Part model, mm, in its own coordinate system. Face numbers are marked on the shaded views. A direction names the side the tool comes from. Give positions to 0.01 mm unless a question says otherwise; leave off trailing zeros. Loops run counter-clockwise (first coordinate to the right, second up) from the corner with the lowest first, then second, coordinate; pieces in that order, holes last. Notation, with made-up numbers: (-22, -17.5) -> (-12, -17.5) arc R19 cw to (-12, 10.5) -> close; hole circle Ø1 at (-21, 45.5). An arc over 180 degrees is marked (long way). One line per question, with ' | ' between items.
```python
from build123d import *

# Parameters (mm, degrees)
F1_DEPTH = 19.05
F2_W     = 44.45
F2_H     = 63.5
F3_DEPTH = 19.05
F4_W     = 44.45
F4_H     = 19.05
F5_DEPTH = 12.7


with BuildPart() as f1:
    # F0 (on Top) → F1 (new body)
    with BuildSketch(Plane.XY):
        Polygon((0, 12.7), (0, 0), (63.5, 0), (63.5, 44.45), (44.45, 44.45), align=None)
    extrude(amount=F1_DEPTH)

    # F2 (on Front) → F3 (join)
    with BuildSketch(Plane.XZ):
        with Locations((41.275, -31.75)):
            Rectangle(F2_W, F2_H)
    extrude(amount=-F3_DEPTH)

    # F4 (on face) → F5 (join)
    with BuildSketch(Plane(origin=(0, 0, -63.5), x_dir=(1, 0, 0), z_dir=(0, 0, -1))):
        Polygon((19.05, 0), (0, 0), (0, -12.8343682736), (44.5106774569, -44.7837524116), (63.5, -44.7837524116), (63.5, -19.05), (19.05, -19.05), align=None)
        with Locations((41.275, -9.525)):
            Rectangle(F4_W, F4_H)
    extrude(amount=F5_DEPTH)


solid = f1.part
```
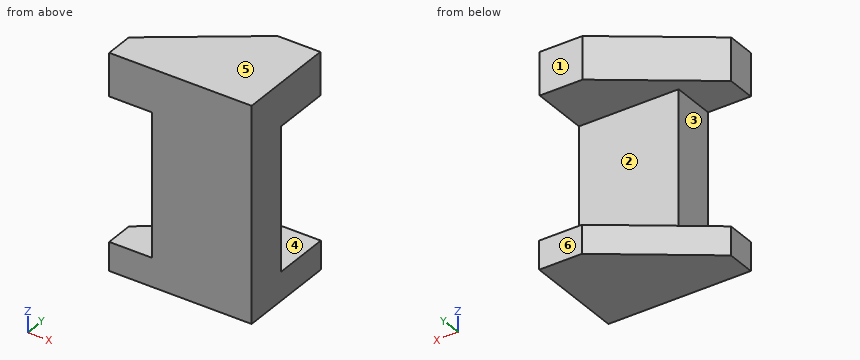
1) Tool access for the marked faces 1, 2 and 3: list every direction of +Z, -Z, +X, -X, +Y, -Y with a clear straight run to the whole face (end or side of a thin tool).
Found:
face 1: +Z, +X, -X, +Y | face 2: +X, -X, +Y | face 3: -X, +Y, -Y
2) Saw through at B-B (x = 11.5). Give the cut face in (y, z), and give its area (3 significant figures).
Found:
outline: (0, -76.2) -> (21.09, -76.2) -> (21.09, -63.5) -> (0, -63.5) -> close; (0, 0) -> (20.91, 0) -> (20.91, 19.05) -> (0, 19.05) -> close | area: 666 mm2
3) Saw through at A-A (y = 41.5). Give the cut face in (x, z).
Found:
outline: (39.94, -76.2) -> (63.5, -76.2) -> (63.5, -63.5) -> (39.94, -63.5) -> close; (40.32, 0) -> (63.5, 0) -> (63.5, 19.05) -> (40.32, 19.05) -> close
4) Pin check, flat tips, straight feed: P1, Ø5.5, axis at y = 11.5, z = -17.5, coming from the -X side; P2, Ø15, axis at x = 51.5, z = 5, coming from the +Y side. Stop position of each tip, or through.
Found:
P1: x = 19.05 | P2: y = 44.45
5) Saw through at D-D (x = 53.5). Give the cut face in (y, z).
Found:
outline: (0, -76.2) -> (44.78, -76.2) -> (44.78, -63.5) -> (19.05, -63.5) -> (19.05, 0) -> (44.45, 0) -> (44.45, 19.05) -> (0, 19.05) -> close
6) Drill centre lines: line 1 (Z direction, x = 5, y = 8); line 2 (X direction, y = 4, z = -46); line 3 (Y direction, x = 43.5, z = -20). Where is each one in solid material? Low to high.
Found:
line 1: -76.2 to -63.5, 0 to 19.05 | line 2: 19.05 to 63.5 | line 3: 0 to 19.05
7) Saw through at C-C (z = 8). Give the cut face in (x, y), and give its area (3 significant figures).
Found:
outline: (0, 0) -> (63.5, 0) -> (63.5, 44.45) -> (44.45, 44.45) -> (0, 12.7) -> close | area: 2,120 mm2
8) Pull direction Z, two halves, no side cores. Call the marked faces 4, 5 and 6: pulls with the +Z half, pulls with the -Z half, needs draft (parallel to the pull), parting line crosses it, or undercut.
Found:
face 4: undercut | face 5: pulls with the +Z half | face 6: needs draft
